from build123d import *

# Parameters (mm, degrees)
F0_W     = 152.4
F0_H     = 67.31
F1_DEPTH = 19.05
F2_R     = 31.75
F3_DEPTH = 15.24
F4_R     = 19.685
F5_DEPTH = 11.43
F6_W     = 19.05
F6_H     = 44.45
F7_DEPTH = 11.43


with BuildPart() as f1:
    # F0 (on Front) → F1 (new body)
    with BuildSketch(Plane.XZ):
        Rectangle(F0_W, F0_H)
    extrude(amount=F1_DEPTH)

    # F2 (on face) → F3 (cut)
    with BuildSketch(Plane.XZ.offset(19.05)):
        Circle(F2_R)
    extrude(amount=-F3_DEPTH, mode=Mode.SUBTRACT)

    # F4 (on face) → F5 (cut)
    with BuildSketch(Plane.XZ.offset(19.05)):
        with Locations((53.34, 0)):
            Circle(F4_R)
    extrude(amount=-F5_DEPTH, mode=Mode.SUBTRACT)

    # F6 (on face) → F7 (cut)
    with BuildSketch(Plane.XZ.offset(19.05)):
        with Locations((-53.34, 0)):
            Rectangle(F6_W, F6_H)
    extrude(amount=-F7_DEPTH, mode=Mode.SUBTRACT)


solid = f1.part
The listing builds one solid part. Answer for the finished solid, in the listing's coordinates (mm). A direction names the side the tool comes from. Round coordinates to 2 decimals unless told otherwise and drop trailing zeros. Loops run counter-clockwise (first coordinate to the right, second up) from the corner with the lowest first, then second, coordinate; pieces in that order, holes last. Notation, with made-up numbers: M -23,41 L 15,41 A8 ccw 15,56 Z; hole C 53,-21 d8. An arc over 180 degrees is marked long. Return JSON: item names as keys, results as strings.
Q1. Find section A-A, the plane y = -14.5. Determine the outline of the cut face in (x, z) (3 decimals), plus the area to 3 significant figures.
Results list:
{"outline": "M -76.2,-33.655 L 76.2,-33.655 L 76.2,33.655 L -76.2,33.655 Z; hole M -62.865,-22.225 L -43.815,-22.225 L -43.815,22.225 L -62.865,22.225 Z; hole C 0,0 d63.5; hole C 53.34,0 d39.37", "area": "5,030 mm2"}
Q2. Find section B-B, the plane x = 53.34. Determine the outline of the cut face in (y, z) (3 decimals), plus the area to 3 significant figures.
Results list:
{"outline": "M -19.05,-33.655 L 0,-33.655 L 0,33.655 L -19.05,33.655 L -19.05,19.685 L -7.62,19.685 L -7.62,-19.685 L -19.05,-19.685 Z", "area": "832 mm2"}
Q3. Which of the six approach directions +Z, -Z, +X, -X, +Y, -Y give full straight-line access (tool end or side, diameter ignored) to faces 4 (the face through (-62.865, -13, 0)), 5 (the face through (-35, -19.05, 0))?
Results list:
{"face 4": "-Y", "face 5": "+Z, -Z, +X, -X, -Y"}
Q4. Find the intervals of material crossed by line 1 along Z through (x, y) = (53.34, -13.25) (3 decimals); line 2 along X through (y, z) = (-8.75, -2) (3 decimals); line 3 along Z through (x, y) = (0, -12.5) (3 decimals), in increasing order. Write a range as from..to.
Results list:
{"line 1": "z = -33.655..-19.685, 19.685..33.655", "line 2": "x = -76.2..-62.865, -43.815..-31.687, 31.687..33.757, 72.923..76.2", "line 3": "z = -33.655..-31.75, 31.75..33.655"}
Q5. Each of these flat-tipped pins is pushed along its axis until it touches: pin 1 Ø19 at (x, z) = (9.5, -3) entering from -Y; pin 2 Ø9.5 at (x, z) = (-58, -9) entering from -Y. Where does it stop, or does it pass through?
Results list:
{"pin 1": "stops at y = -3.81", "pin 2": "stops at y = -7.62"}
Q6. Find section C-C, the plane y = -6. Determine the outline of the cut face in (x, z) (3 decimals).
Results list:
{"outline": "M -76.2,-33.655 L 76.2,-33.655 L 76.2,33.655 L -76.2,33.655 Z; hole C 0,0 d63.5"}
Q7. Find section D-D, the plane z = -10.5. Determine the outline of the cut face in (x, y) (3 decimals), plus the area to 3 significant figures.
Results list:
{"outline": "M -76.2,-19.05 L -62.865,-19.05 L -62.865,-7.62 L -43.815,-7.62 L -43.815,-19.05 L -29.964,-19.05 L -29.964,-3.81 L 29.964,-3.81 L 29.964,-19.05 L 36.689,-19.05 L 36.689,-7.62 L 69.991,-7.62 L 69.991,-19.05 L 76.2,-19.05 L 76.2,0 L -76.2,0 Z", "area": "1,390 mm2"}
Q8. The mould has two halves that part along X. Classify faces 1 (the face through (72.116, -13.415, 5.913)), 2 (the face through (-1, 0, 0)), 3 (the face through (-76.2, -9, 0)): released by +X, released by -X, zero draft, split by the parting line, or undercut.
Results list:
{"face 1": "undercut", "face 2": "zero draft", "face 3": "released by -X"}
